from build123d import *

# Parameters (mm, degrees)
F1_DEPTH = 3
F3_D     = 1
F4_R     = 1.49999


# Not quite as in the source:
# - a fillet or chamfer is up to 0.001 mm smaller than in the source, because OpenCascade refuses the exact size
# - ends of sketch curves that miss each other by under 0.0002 mm in the source are joined


with BuildPart() as f1:
    # F0 (on Right) → F1 (new body)
    with BuildSketch(Plane.YZ):
        with BuildLine():
            Line((-45, 3), (-45, 0))
            Line((-45, 0), (45, 0))
            ThreePointArc((45, 0), (59.1421356237, -5.8578643763), (65, -20))
            ThreePointArc((65, -20), (66.5000000156, -21.499999553), (68, -19.999999553))
            ThreePointArc((68, -19.999999553), (61.2634559673, -3.7365440327), (45, 3))
            Line((45, 3), (-45, 3))
        make_face()
    extrude(amount=F1_DEPTH)

    # F3 (through all)
    with Locations(Plane(origin=(0, 0, 0), x_dir=(1, 0, 0), z_dir=(0, 0, -1))):
        with Locations((1.5, 43)):
            Hole(F3_D / 2)

    # F4 (radius 1.5 in the source; OpenCascade refuses exactly that, so slightly less here)
    f4_edges = [f1.edges().sort_by_distance(p)[0] for p in [
        (3, -45, 1.5),
        (0, -45, 1.5),
    ]]
    fillet(f4_edges, radius=F4_R)


solid = f1.part
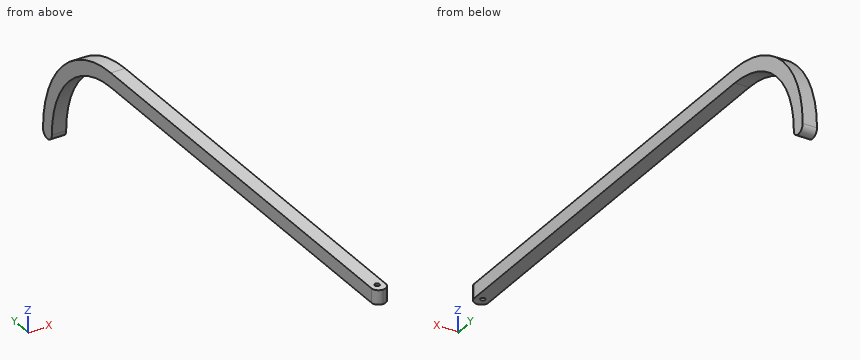
For this review, take the finished solid that the model builds, in its own axes (mm). Coordinates: 2 decimals unless noted, no trailing zeros. Write each loop counter-clockwise with the first axis right and the second up, starting at its lowest first coordinate (ties: lowest second). Pieces come first, ordered by that corner, then holes. Notation, with made-up numbers: (21.5, 1) -> (70.5, 1) arc R27 ccw to (70.5, 17) -> close; hole circle Ø2 at (-12.75, -11). An arc over 180 degrees is marked (long way). Write each question's results on one line, items separated by ' | '. Start each with the question number.
1) Consider section B-B (z = -13.25). Write out the cut boundary in (x, y), plus the area to 3 significant figures.
2) Wall thickness on L1, parallel to X at y = -43, z = 1.9; L2, parallel to Z at x = 1.2, y = -1.5; L3, parallel to Y at x = 1.4, z = 0.25: over which ranges is each line inside the solid? List them lowest first. Write a range as [from, to].
3) Consider section A-A (y = 39). Write out the cut boundary in (x, z), plus the area to 3 significant figures.
Geometry says:
1) outline: (0, 63.83) -> (3, 63.83) -> (3, 66.99) -> (0, 66.99) -> close | area: 9.48 mm^2
2) L1: [0, 1], [2, 3] | L2: [0, 3] | L3: [-45, -43.49], [-42.51, 55.91]
3) outline: (0, 0) -> (3, 0) -> (3, 3) -> (0, 3) -> close | area: 9.00 mm^2
